Drawing for the job (mm, zero at the part's lowest x, y, z). A direction names the side the tool comes from. Give positions to 0.01 mm unless a question says otherwise; leave off trailing zeros. Loops run counter-clockwise (first coordinate to the right, second up) from the corner with the lowest first, then second, coordinate; pieces in that order, holes last. Notation, with made-up numbers: (-2.75, 9) -> (34.25, 9) arc R34 ccw to (34.25, 45) -> close; hole circle Ø10 at (-39.75, -10). An arc over 180 degrees is marked (long way). Answer in a Markdown table with one row per item. Add a question column.
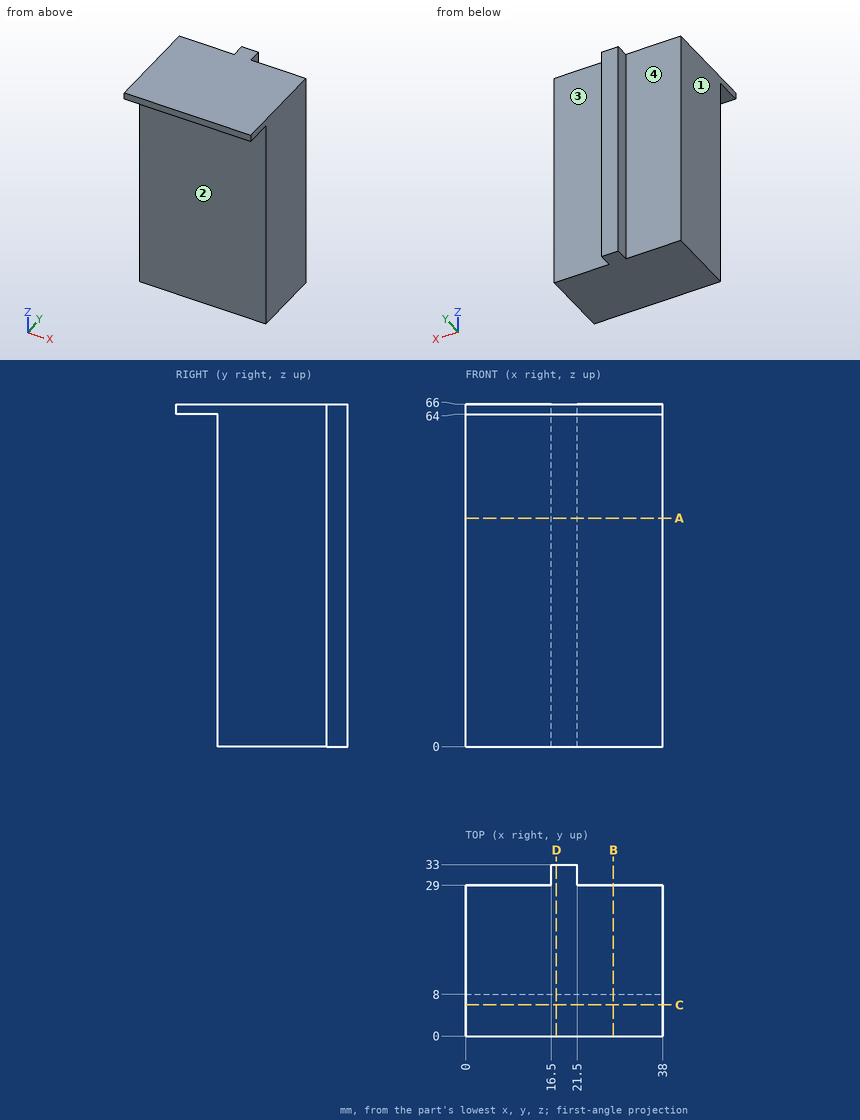
(1) Saw through at D-D, the plane x = 17.5. List the corners of the cut face in (y, z), then the cut area to 3 significant figures.
(2) Flat gauge pins, fed straight in: pin 1 Ø19 at (x, z) = (17.5, 32.5) entering from -Y; pin 2 Ø3 at (x, z) = (11, 31.5) entering from +Y; pin 3 Ø2 at (y, z) = (32, 25) entering from +X. Where does each tip first touch, or does it go through?
(3) Saw through at B-B, the plane x = 28.5. List the corners of the cut face in (y, z), then the cut area to 3 significant figures.
(4) 3-axis set-ups, long thin cutter, end or side, ignore diameter. For the marked faces 1, 2, 3 and 4: which of +Z, -Z, +X, -X, +Y, -Y reach the whole face in a straight line?
(5) Saw through at C-C, the plane y = 6. List the corners of the cut face in (x, z).
(6) Saw through at A-A, the plane z = 44. List the corners of the cut face in (x, y), then the cut area to 3 significant figures.
(7) Wall check: line 1 along Y through (x, z) = (8.5, 37); line 2 along X through (y, z) = (31, 25); line 3 along Z through (x, y) = (17, 5). Give the ranges that are in metal, low to high. Write a range as from..to.
Worked answers:
| question | item | result |
|---|---|---|
| 1 | outline | (0, 64) -> (8, 64) -> (8, 0) -> (33, 0) -> (33, 66) -> (0, 66) -> close |
| 1 | area | 1,670 mm^2 |
| 2 | pin 1 | y = 8 |
| 2 | pin 2 | y = 29 |
| 2 | pin 3 | x = 21.5 |
| 3 | outline | (0, 64) -> (8, 64) -> (8, 0) -> (29, 0) -> (29, 66) -> (0, 66) -> close |
| 3 | area | 1,400 mm^2 |
| 4 | face 1 | +Z, -Z, -X, +Y, -Y |
| 4 | face 2 | -Z, +X, -X, -Y |
| 4 | face 3 | +Z, -Z, +X, +Y |
| 4 | face 4 | +Z, -Z, -X, +Y |
| 5 | outline | (0, 64) -> (38, 64) -> (38, 66) -> (0, 66) -> close |
| 6 | outline | (0, 8) -> (38, 8) -> (38, 29) -> (21.5, 29) -> (21.5, 33) -> (16.5, 33) -> (16.5, 29) -> (0, 29) -> close |
| 6 | area | 818 mm^2 |
| 7 | line 1 | 8..29 |
| 7 | line 2 | 16.5..21.5 |
| 7 | line 3 | 64..66 |
